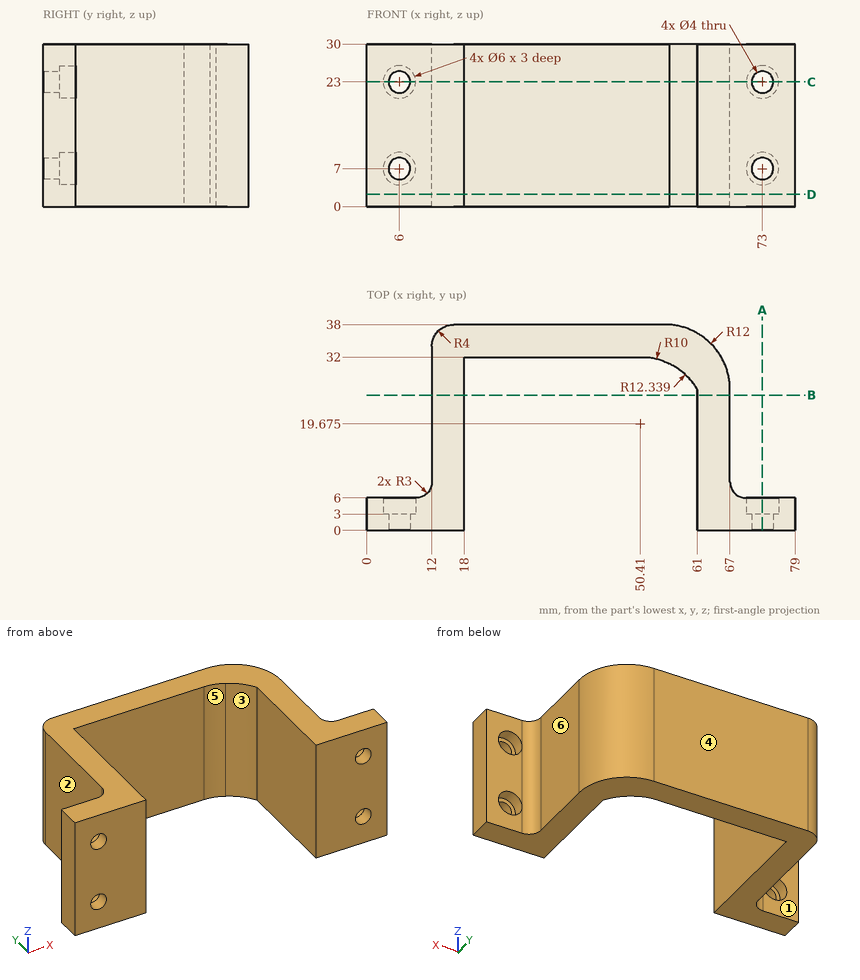
Print and shaded views of the part. All mm, measured from the part's lowest x, y and z. A direction names the side the tool comes from. Coordinates: 2 decimals unless noted, no trailing zeros. Loops run counter-clockwise (first coordinate to the right, second up) from the corner with the lowest first, then second, coordinate; pieces in that order, holes last. Notation, with made-up numbers: (54.5, 8) - (112.5, 8) arc R22 cw to (112.5, 36) - close; hole circle Ø3 at (64, 33). An arc over 180 degrees is marked (long way). Write item = value, one per line. Start each with the question number.
Item 1: Cut at D-D, the plane z = 2.25. Give the cut face in (x, y) (1 decimal), and give its area (3 significant figures).
Item 2: Wall check: L1, parallel to Z at x = 6, y = 4; L2, parallel to Z at x = 6, y = 1; L3, parallel to X at y = 1.55, z = 7. Give the ranges that are in metal, low to high. Write a range as from..to.
Item 3: Cut at A-A, the plane x = 73. Give the cut face in (y, z).
Item 4: Cut at C-C, the plane z = 23. State how many separate pieces and enclosed holes the cut face has, and give its area (3 significant figures).
Item 5: 3-axis set-ups, long thin cutter, end or side, ignore diameter. For the marked faces 4, 5 and 6: which of +Z, -Z, +X, -X, +Y, -Y reach the whole face in a straight line?
Item 6: Mould opens along X. For the marked faces 1, 2 and 3 say: released by +X, released by -X, zero draft, split by the parting line, or undercut.
Item 7: Flat gauge pins, fed straight in: pin 1 Ø6 at (y, z) = (20.5, 23) entering from +X; pin 2 Ø6.5 at (x, z) = (73, 22.5) entering from +Y; pin 3 Ø12 at (y, z) = (13, 19.5) entering from +X (1 decimal). Where does each tip first touch, or does it go through?
Item 8: Cut at B-B, the plane y = 25. Give the cut face in (x, z).
The answers:
q1.outline = (0, 0) - (18, 0) - (18, 32) - (51, 32) arc R10 cw to (55.8, 30.8) arc R12.3 cw to (61, 26) - (61, 0) - (79, 0) - (79, 6) - (70, 6) arc R3 cw to (67, 9) - (67, 26) arc R12 ccw to (55, 38) - (16, 38) arc R4 ccw to (12, 34) - (12, 9) arc R3 cw to (9, 6) - (0, 6) - close
q1.area = 846 mm2
q2.L1 = 0..4, 10..20, 26..30
q2.L2 = 0..5, 9..21, 25..30
q2.L3 = 0..4, 8..18, 61..71, 75..79
q3.outline = (0, 0) - (6, 0) - (6, 4) - (3, 4) - (3, 5) - (0, 5) - close; (0, 9) - (3, 9) - (3, 10) - (6, 10) - (6, 20) - (3, 20) - (3, 21) - (0, 21) - close; (0, 25) - (3, 25) - (3, 26) - (6, 26) - (6, 30) - (0, 30) - close
q4.separate_pieces = 3
q4.enclosed_holes = 0
q4.area = 786 mm2
q5.face_4 = +Z, -Z, +X, -X, +Y
q5.face_5 = +Z, -Z, -Y
q5.face_6 = +Z, -Z, +X, +Y
q6.face_1 = zero draft
q6.face_2 = released by -X
q6.face_3 = undercut
q7.pin_1 = 67
q7.pin_2 = 6.01
q7.pin_3 = 67.8
q8.outline = (12, 0) - (18, 0) - (18, 30) - (12, 30) - close; (61, 0) - (67, 0) - (67, 30) - (61, 30) - close
